from build123d import *

# Parameters (mm, degrees)
AUFSATZ_LINEAR_AUSTRAGEN1_DEPTH   = 6
AUFSATZ_LINEAR_AUSTRAGEN1_2_DEPTH = 6
SKIZZE4_W                         = 9.24
SKIZZE4_H                         = 10.88
AUFSATZ_LINEAR_AUSTRAGEN2_DEPTH   = 2
SKIZZE3_R                         = 1.65
SCHNITT_LINEAR_AUSTRAGEN1_DEPTH   = 10.88
FASE1_SIZE                        = 0.5


with BuildPart() as part:
    # Skizze1 → Aufsatz-Linear austragen1 (new body)
    with BuildSketch(Plane.XY):
        Polygon((0, 0), (0, 9.44), (0, 10.88), (-6, 10.88), (-6, 0), align=None)
    extrude(amount=AUFSATZ_LINEAR_AUSTRAGEN1_DEPTH)



with BuildPart() as body_2:
    # Skizze1 → Aufsatz-Linear austragen1 2 (new body)
    with BuildSketch(Plane.XY):
        with BuildLine():
            Line((-7.05, 10.19), (-7.05, 10.69))
            ThreePointArc((-7.05, 10.69), (-7.105649712, 10.824350288), (-7.24, 10.88))
            Line((-7.24, 10.88), (-9.24, 10.88))
            Line((-9.24, 10.88), (-9.24, 0))
            Line((-9.24, 0), (-7.24, 0))
            ThreePointArc((-7.24, 0), (-7.105649712, 0.055649712), (-7.05, 0.19))
            Line((-7.05, 0.19), (-7.05, 0.69))
            ThreePointArc((-7.05, 0.69), (-7.105649712, 0.824350288), (-7.24, 0.88))
            ThreePointArc((-7.24, 0.88), (-7.8, 1.44), (-7.24, 2))
            ThreePointArc((-7.24, 2), (-7.105649712, 2.055649712), (-7.05, 2.19))
            Line((-7.05, 2.19), (-7.05, 2.69))
            ThreePointArc((-7.05, 2.69), (-7.105649712, 2.824350288), (-7.24, 2.88))
            ThreePointArc((-7.24, 2.88), (-7.8, 3.44), (-7.24, 4))
            ThreePointArc((-7.24, 4), (-7.105649712, 4.055649712), (-7.05, 4.19))
            Line((-7.05, 4.19), (-7.05, 4.69))
            ThreePointArc((-7.05, 4.69), (-7.105649712, 4.824350288), (-7.24, 4.88))
            ThreePointArc((-7.24, 4.88), (-7.8, 5.44), (-7.24, 6))
            ThreePointArc((-7.24, 6), (-7.105649712, 6.055649712), (-7.05, 6.19))
            Line((-7.05, 6.19), (-7.05, 6.69))
            ThreePointArc((-7.05, 6.69), (-7.105649712, 6.824350288), (-7.24, 6.88))
            ThreePointArc((-7.24, 6.88), (-7.8, 7.44), (-7.24, 8))
            ThreePointArc((-7.24, 8), (-7.105649712, 8.055649712), (-7.05, 8.19))
            Line((-7.05, 8.19), (-7.05, 8.69))
            ThreePointArc((-7.05, 8.69), (-7.105649712, 8.824350288), (-7.24, 8.88))
            ThreePointArc((-7.24, 8.88), (-7.8, 9.44), (-7.24, 10))
            ThreePointArc((-7.24, 10), (-7.105649712, 10.055649712), (-7.05, 10.19))
        make_face()
    extrude(amount=AUFSATZ_LINEAR_AUSTRAGEN1_2_DEPTH)


with BuildPart() as part_1:
    add(part.part)

    add(body_2.part)  # Aufsatz-Linear austragen2 merges body 2
    # Skizze4 → Aufsatz-Linear austragen2 (add)
    with BuildSketch(Plane(origin=(0, 0, 0), x_dir=(-1, 0, 0), z_dir=(0, 0, -1))):
        with Locations((4.62, 5.44)):
            Rectangle(SKIZZE4_W, SKIZZE4_H)
    extrude(amount=AUFSATZ_LINEAR_AUSTRAGEN2_DEPTH)

    # Skizze3 → Schnitt-Linear austragen1 (cut)
    with BuildSketch(Plane(origin=(0, 10.88, 0), x_dir=(1, 0, 0), z_dir=(0, 1, 0))):
        with Locations(Location((-3, -3, 0), (0, 0, 180))):
            Circle(SKIZZE3_R)
    extrude(amount=-SCHNITT_LINEAR_AUSTRAGEN1_DEPTH, mode=Mode.SUBTRACT)

    # Fase1
    fase1_edges = [part_1.edges().sort_by_distance(p)[0] for p in [
        (-6, 10.88, 3),
        (-6, 0, 3),
    ]]
    chamfer(fase1_edges, length=FASE1_SIZE)


solid = part_1.part
Work out the finished part from the listing and answer in its coordinate system (mm). A direction names the side the tool comes from. Give positions to 0.01 mm unless a question says otherwise; leave off trailing zeros. Order: outer loops, then holes, each group sorted by start corner. A loop starts at its lowest first (then second) coordinate and runs counter-clockwise, first axis right, second up. Notation, with made-up numbers: (-15, 10) - (25, 10) arc R15 ccw to (25, 33) - close; hole circle Ø10 at (2.5, 37). An arc over 180 degrees is marked (long way). Answer as CSV lines item,"result". Start each with the question number.
Q1. The part is cut by section C-C (x = -2.5). Write down the section's boundary in (y, z).
Q2. For faces 1 (the face through (0, 5, 2)), 2 (the face through (-6, 6, 3)), 3 (the face through (-7.8, 9.4, 3)), determine the directions among +Z, -Z, +X, -X, +Y, -Y from which every point of the face is accessible in a straight line to the end or side of a thin tool.
Q3. Find the intervals of material crossed by L1, parallel to X at y = 1, z = 1.75; L2, parallel to Z at x = -3, y = 3; L3, parallel to X at y = 10.5, z = 3.75, in increasing order. Write a range as [from, to].
Q4. The mould has two halves that part along Z. Classify faces 4 (the face through (-3, 6, 6)), 5 (the face through (-5, 6, -2)), 6 (the face through (-2.785, 5.516, 4.636)), 7 (the face through (-7.8, 1.4, 3)): +Z half, -Z half, draft (parallel to the pull), parting line (faces both ways), or undercut.
Q5. Given pin 1 Ø0.6 at (y, z) = (10.5, 2.5) entering from +X; pin 2 Ø3 at (x, z) = (-3, 3) entering from -Y, each flat-ended and moving along its own axis, determine where each tip first touches the part or whether it passes through.
Q6. The part is cut by section D-D (z = 3). Give the number of separate pieces and of enclosed holes in the cut face, then the cut area to 3 significant figures.
Q7. The part is cut by section B-B (y = 7.44). Write down the section's boundary in (x, z), then the cut area to 3 significant figures.
Check result:
1,outline,"(0, -2) - (10.88, -2) - (10.88, 1.43) - (0, 1.43) - close; (0, 4.57) - (10.88, 4.57) - (10.88, 6) - (0, 6) - close"
2,face 1,"+Z, -Z, +X, +Y, -Y"
2,face 2,"+Z, +Y, -Y"
2,face 3,"+Z"
3,L1,"x = [-9.24, -7.59], [-6, -4.08], [-1.92, 0]"
3,L2,"z = [-2, 1.35], [4.65, 6]"
3,L3,"x = [-9.24, -7.05], [-5.88, -4.47], [-1.53, 0]"
4,face 4,"+Z half"
4,face 5,"-Z half"
4,face 6,"undercut"
4,face 7,"draft"
5,pin 1,"stops at x = 0"
5,pin 2,"passes through"
6,separate pieces,"3"
6,enclosed holes,"0"
6,area,"49.3 mm²"
7,outline,"(-9.24, -2) - (0, -2) - (0, 6) - (-6, 6) - (-6, 0) - (-7.8, 0) - (-7.8, 6) - (-9.24, 6) - close; hole circle Ø3.3 at (-3, 3)"
7,area,"54.6 mm²"
